```python
from build123d import *

# Parameters (mm, degrees)
SKETCH1_R           = 25.4
BOSS_EXTRUDE1_DEPTH = 3.175
SKETCH2_R           = 22.225
BOSS_EXTRUDE2_DEPTH = 12.7
SKETCH3_R           = 9.525
CUT_EXTRUDE1_DEPTH  = 16.875
CHAMFER1_SIZE       = 1.5
CHAMFER2_SIZE       = 1


with BuildPart() as part:
    # Sketch1 → Boss-Extrude1 (new body)
    with BuildSketch(Plane(origin=(0, 0, 0), x_dir=(0, 0, -1), z_dir=(1, 0, 0))):
        Circle(SKETCH1_R)
    extrude(amount=BOSS_EXTRUDE1_DEPTH)

    # Sketch2 → Boss-Extrude2 (add)
    with BuildSketch(Plane(origin=(3.175, 0, 0), x_dir=(0, 0, -1), z_dir=(1, 0, 0))):
        Circle(SKETCH2_R)
    extrude(amount=BOSS_EXTRUDE2_DEPTH)

    # Sketch3 → Cut-Extrude1 (cut, through all)
    with BuildSketch(Plane.ZY):
        Circle(SKETCH3_R)
    extrude(amount=-CUT_EXTRUDE1_DEPTH, mode=Mode.SUBTRACT)

    # Chamfer1
    chamfer1_edges = [part.edges().sort_by_distance(p)[0] for p in [
        (3.175, 0, 25.4),
    ]]
    chamfer(chamfer1_edges, length=CHAMFER1_SIZE)

    # Chamfer2
    chamfer2_edges = [part.edges().sort_by_distance(p)[0] for p in [
        (15.875, 0, 22.225),
    ]]
    chamfer(chamfer2_edges, length=CHAMFER2_SIZE)


solid = part.part
```
Design review of the part built by this model. Coordinates are the model's own, in mm. A direction names the side the tool comes from. Coordinates: 2 decimals unless noted, no trailing zeros. Loops run counter-clockwise (first coordinate to the right, second up) from the corner with the lowest first, then second, coordinate; pieces in that order, holes last. Notation, with made-up numbers: M -21.5,0 L 10.5,0 A18 ccw 10.5,25 Z; hole C 27,-3.75 d4. An arc over 180 degrees is marked long. One line per question, with ' | ' between items.
(1) Draft analysis for pull direction Z (two halves, no side actions). For faces 3 (the face through (15.875, -4, -9)), 4 (the face through (0.826, -24.796, 5.506)), 5 (the face through (7.826, -5.796, -7.559)), state which applies: released by +Z, released by -Z, zero draft, split by the parting line, or undercut.
Filled in:
face 3: zero draft | face 4: split by the parting line | face 5: undercut
(2) We need section C-C (x = 4.5). Give the boundary of the cut face in (y, z) (3 decimals).
Filled in:
outline: C 0,0 d44.45; hole C 0,0 d19.05
(3) Wall thickness on probe 1 along Y at (x, z) = (9.75, 0) (3 decimals); probe 2 along Y at (x, z) = (11, 6); probe 3 along Y at (x, z) = (6.75, 17.5): over which ranges is each line inside the solid? List them lowest first.
Filled in:
probe 1: y = -22.225 to -9.525, 9.525 to 22.225 | probe 2: y = -21.4 to -7.4, 7.4 to 21.4 | probe 3: y = -13.7 to 13.7
(4) For pin 1 Ø1 at (x, y) = (5, 8.5) entering from +Z; pin 2 Ø22 at (y, z) = (0, 0) entering from -X; pin 3 Ø8 at (x, y) = (14, 7.5) entering from -Z; pin 4 Ø4 at (x, z) = (11.5, -12.5) entering from -Y, all flat-tipped, find the tip position at first contact; note any pin that passes through.
Filled in:
pin 1: stops at z = 20.74 | pin 2: stops at x = 0 | pin 3: stops at z = -21.95 | pin 4: stops at y = -19.59
(5) Machinability: for faces 1 (the face through (8.943, 6.676, -21.199)), 2 (the face through (0, 0, -11)), which of the approach directions +Z, -Z, +X, -X, +Y, -Y give a long, thin tool a straight path to every point of the face, cutting with its end or side? Answer none if there is none.
Filled in:
face 1: +X | face 2: +Z, -Z, -X, +Y, -Y
(6) We need section A-A (y = 0). Give the boundary of the cut face in (x, z) (3 decimals), and give its area (3 significant figures).
Filled in:
outline: M 0,-25.4 L 1.675,-25.4 L 3.175,-23.9 L 3.175,-22.225 L 14.875,-22.225 L 15.875,-21.225 L 15.875,-9.525 L 0,-9.525 Z; M 0,9.525 L 15.875,9.525 L 15.875,21.225 L 14.875,22.225 L 3.175,22.225 L 3.175,23.9 L 1.675,25.4 L 0,25.4 Z | area: 420 mm^2
